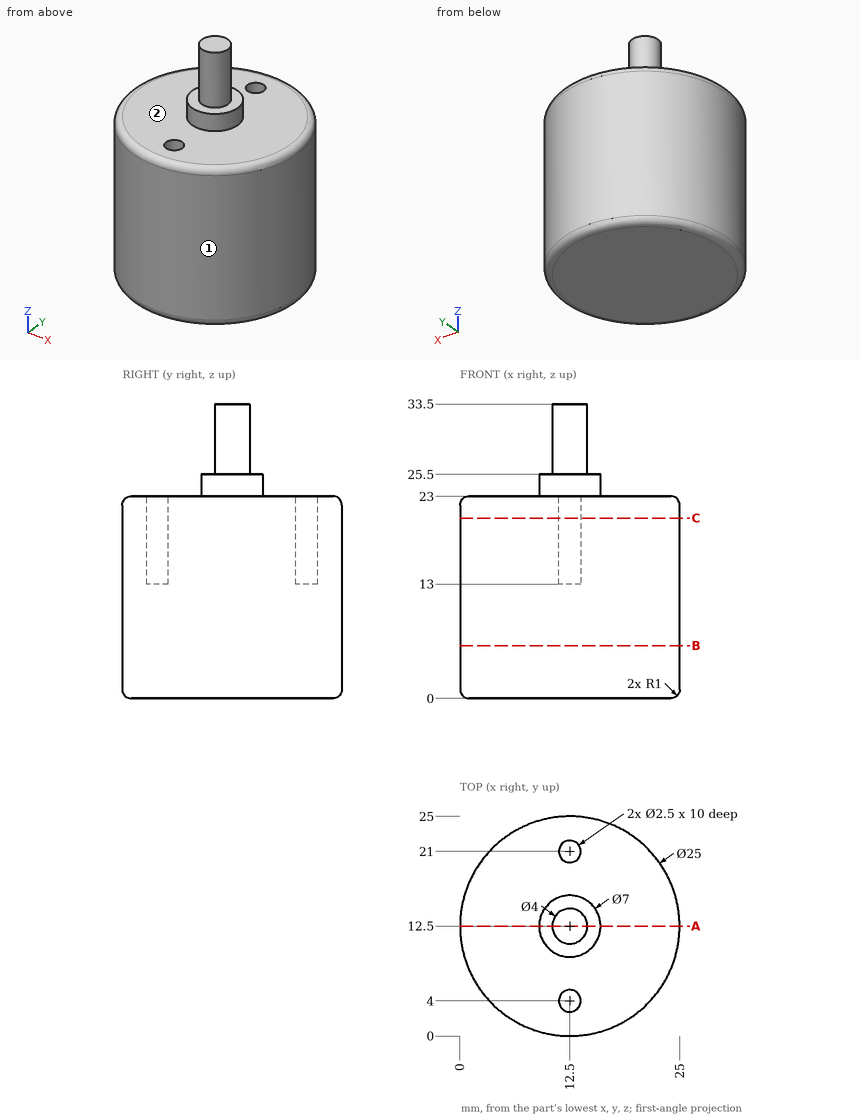
Print and shaded views of the part. All mm, measured from the part's lowest x, y and z. A direction names the side the tool comes from. Coordinates: 2 decimals unless noted, no trailing zeros. Order: outer loops, then holes, each group sorted by start corner. A loop starts at its lowest first (then second) coordinate and runs counter-clockwise, first axis right, second up. Notation, with made-up numbers: M 52,34 L 85,34 A13 ccw 85,52 Z; hole C 13,2.5 d3. An arc over 180 degrees is marked long. One line per question, with ' | ' between items. Start each with the question number.
Q1. Probe L1, parallel to Y at x = 12.5, z = 16.5; L2, parallel to Z at x = 6.75, y = 16.75; L3, parallel to X at y = 12.75, z = 22. List the from-to ranges inside material, lowest first. Write a range as from..to.
Q2. Saw through at C-C (z = 20.5). List the corners of the cut face in (x, y), then the cut area to 3 significant figures.
Q3. Saw through at A-A (y = 12.5). List the corners of the cut face in (x, z), then the cut area to 3 significant figures.
Q4. Saw through at B-B (z = 6). List the corners of the cut face in (x, y), then the cut area to 3 significant figures.
Q5. Flat gauge pins, fed straight in: pin 1 Ø3 at (x, z) = (20, 14.5) entering from -Y; pin 2 Ø1.2 at (x, y) = (12.5, 21.5) entering from +Z; pin 3 Ø1.5 at (x, z) = (15.5, 23.5) entering from -Y. Where does each tip first touch, or does it go through?
Q6. 3-axis set-ups, long thin cutter, end or side, ignore diameter. For the marked faces 1 and 2: which of +Z, -Z, +X, -X, +Y, -Y reach the whole face in a straight line?
Check values:
1) L1: y = 0..2.75, 5.25..19.75, 22.25..25 | L2: z = 0..23 | L3: x = 0..25
2) outline: C 12.5,12.5 d25; hole C 12.5,4 d2.5; hole C 12.5,21 d2.5 | area: 481 mm2
3) outline: M 0,1 A1 ccw 1,0 L 24,0 A1 ccw 25,1 L 25,22 A1 ccw 24,23 L 16,23 L 16,25.5 L 14.5,25.5 L 14.5,33.5 L 10.5,33.5 L 10.5,25.5 L 9,25.5 L 9,23 L 1,23 A1 ccw 0,22 Z | area: 624 mm2
4) outline: C 12.5,12.5 d25 | area: 491 mm2
5) pin 1: stops at y = 1.53 | pin 2: stops at z = 13 | pin 3: stops at y = 0.7
6) face 1: +Z, -Z | face 2: +Z
